from build123d import *

# Parameters (mm, degrees)
SKETCH1_R             = 30
BOSS_EXTRUDE1_DEPTH   = 500
BOSS_EXTRUDE1_2_DEPTH = 500
BOSS_EXTRUDE1_3_DEPTH = 500
BOSS_EXTRUDE1_4_DEPTH = 500
SKETCH2_W             = 500
SKETCH2_H             = 500
BOSS_EXTRUDE2_DEPTH   = 100
SKETCH3_W             = 400
SKETCH3_H             = 400
BOSS_EXTRUDE3_DEPTH   = 100
SKETCH4_W             = 300
SKETCH4_H             = 300
BOSS_EXTRUDE4_DEPTH   = 100
SKETCH5_R             = 50
BOSS_EXTRUDE5_DEPTH   = 100
SKETCH6_R             = 40
CUT_EXTRUDE1_DEPTH    = 40


with BuildPart() as part:
    # Sketch1 → Boss-Extrude1 (new body)
    with BuildSketch(Plane(origin=(0, 0, 0), x_dir=(1, 0, 0), z_dir=(0, 1, 0))):
        with Locations(Location((-190, -190, 0), (0, 0, 270))):
            Circle(SKETCH1_R)
    extrude(amount=BOSS_EXTRUDE1_DEPTH)



with BuildPart() as body_2:
    # Sketch1 → Boss-Extrude1 2 (new body)
    with BuildSketch(Plane(origin=(0, 0, 0), x_dir=(1, 0, 0), z_dir=(0, 1, 0))):
        with Locations(Location((-190, 190, 0), (0, 0, 270))):
            Circle(SKETCH1_R)
    extrude(amount=BOSS_EXTRUDE1_2_DEPTH)


with BuildPart() as body_3:
    # Sketch1 → Boss-Extrude1 3 (new body)
    with BuildSketch(Plane(origin=(0, 0, 0), x_dir=(1, 0, 0), z_dir=(0, 1, 0))):
        with Locations(Location((190, 190, 0), (0, 0, 270))):
            Circle(SKETCH1_R)
    extrude(amount=BOSS_EXTRUDE1_3_DEPTH)


with BuildPart() as body_4:
    # Sketch1 → Boss-Extrude1 4 (new body)
    with BuildSketch(Plane(origin=(0, 0, 0), x_dir=(1, 0, 0), z_dir=(0, 1, 0))):
        with Locations(Location((190, -190, 0), (0, 0, 270))):
            Circle(SKETCH1_R)
    extrude(amount=BOSS_EXTRUDE1_4_DEPTH)


with BuildPart() as part_1:
    add(part.part)

    add(body_2.part)  # Boss-Extrude2 merges body 2

    add(body_3.part)  # Boss-Extrude2 merges body 3

    add(body_4.part)  # Boss-Extrude2 merges body 4
    # Sketch2 → Boss-Extrude2 (add)
    with BuildSketch(Plane(origin=(0, 500, 0), x_dir=(1, 0, 0), z_dir=(0, 1, 0))):
        Rectangle(SKETCH2_W, SKETCH2_H)
    extrude(amount=BOSS_EXTRUDE2_DEPTH)

    # Sketch3 → Boss-Extrude3 (add)
    with BuildSketch(Plane(origin=(0, 600, 0), x_dir=(1, 0, 0), z_dir=(0, 1, 0))):
        Rectangle(SKETCH3_W, SKETCH3_H)
    extrude(amount=BOSS_EXTRUDE3_DEPTH)

    # Sketch4 → Boss-Extrude4 (add)
    with BuildSketch(Plane(origin=(0, 700, 0), x_dir=(1, 0, 0), z_dir=(0, 1, 0))):
        Rectangle(SKETCH4_W, SKETCH4_H)
    extrude(amount=BOSS_EXTRUDE4_DEPTH)

    # Sketch5 → Boss-Extrude5 (add)
    with BuildSketch(Plane(origin=(0, 800, 0), x_dir=(1, 0, 0), z_dir=(0, 1, 0))):
        with Locations(Location((0, 0, 0), (0, 0, 270))):
            Circle(SKETCH5_R)
    extrude(amount=BOSS_EXTRUDE5_DEPTH)

    # Sketch6 → Cut-Extrude1 (cut)
    with BuildSketch(Plane(origin=(0, 900, 0), x_dir=(1, 0, 0), z_dir=(0, 1, 0))):
        with Locations(Location((0, 0, 0), (0, 0, 270))):
            Circle(SKETCH6_R)
    extrude(amount=-CUT_EXTRUDE1_DEPTH, mode=Mode.SUBTRACT)


solid = part_1.part
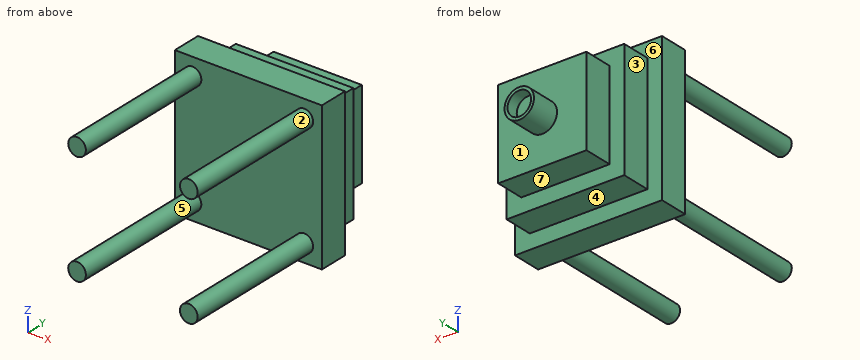
Can you work these out from the model? Positions are in its coordinate system, mm. Face numbers are marked on the shaded views. A direction names the side the tool comes from. Coordinates: 2 decimals unless noted, no trailing zeros. Loops run counter-clockwise (first coordinate to the right, second up) from the corner with the lowest first, then second, coordinate; pieces in that order, holes last. Notation, with made-up numbers: M 48.25,13 L 60.25,13 A22 ccw 60.25,25 Z; hole C -18.75,35.5 d11. An arc over 180 degrees is marked long. Return JSON: item names as keys, results as strings. Group by question number.
Item 1: On a 3-axis mill with a long thin cutter (end or side, diameter ignored), from which of +Z, -Z, +X, -X, +Y, -Y can I reach the whole of each face in a straight line? I mean the marked faces 1, 2, 3 and 4. Say none if no direction works.
Item 2: If I drill on L1, parallel to X at y = 880.5, z = 0; L2, parallel to Y at x = 156.5, z = 11; L3, parallel to Y at x = 90, z = 1.5, over which ranges is the centre line in solid material (lowest first)? Write a range as from..to.
Item 3: Imagine slicing it at C-C (y = 93). Please give me the cut outline in (x, z), and give its area (3 significant figures).
Item 4: Imagine slicing it at D-D (y = 774.5). Please give me the cut outline in (x, z).
Item 5: I'm going to push flat-ended pins straight in: pin 1 Ø1.5 at (y, z) = (677.5, -90) entering from -X; pin 2 Ø1 at (x, z) = (162.5, -142.5) entering from +Y; pin 3 Ø4 at (x, y) = (-23, 691.5) entering from -Z. Where does each tip first touch, or does it pass through?
Item 6: Imagine slicing it at B-B (x = -190). Please give me the cut outline in (y, z), and give its area (3 significant figures).
Item 7: Thinking about a two-plate mould opening in Z: for the marked faces 5, 6 and 7, which applies, released by +Z, released by -Z, zero draft, split by the parting line, or undercut?
Item 8: Imagine slicing it at A-A (z = 0). Please give me the cut outline in (x, y).
Verdict:
{
 "1": {"face 1": "+Y", "face 2": "-Y", "face 3": "+Z, -Z, -X, +Y", "face 4": "-Z, +X, -X, +Y"},
 "2": {"L1": "x = -50..-40, 40..50", "L2": "y = 500..700", "L3": "y = 500..800"},
 "3": {"outline": "C -190,-190 d60; C -190,190 d60; C 190,-190 d60; C 190,190 d60", "area": "11,300 mm^2"},
 "4": {"outline": "M -150,-150 L 150,-150 L 150,150 L -150,150 Z"},
 "5": {"pin 1": "stops at x = -200", "pin 2": "stops at y = 700", "pin 3": "stops at z = -200"},
 "6": {"outline": "M 0,-220 L 500,-220 L 500,-250 L 600,-250 L 600,-200 L 700,-200 L 700,200 L 600,200 L 600,250 L 500,250 L 500,220 L 0,220 L 0,160 L 500,160 L 500,-160 L 0,-160 Z", "area": "150,000 mm^2"},
 "7": {"face 5": "undercut", "face 6": "zero draft", "face 7": "released by -Z"},
 "8": {"outline": "M -250,500 L 250,500 L 250,600 L 200,600 L 200,700 L 150,700 L 150,800 L 50,800 L 50,900 L 40,900 L 40,860 L -40,860 L -40,900 L -50,900 L -50,800 L -150,800 L -150,700 L -200,700 L -200,600 L -250,600 Z"}
}
